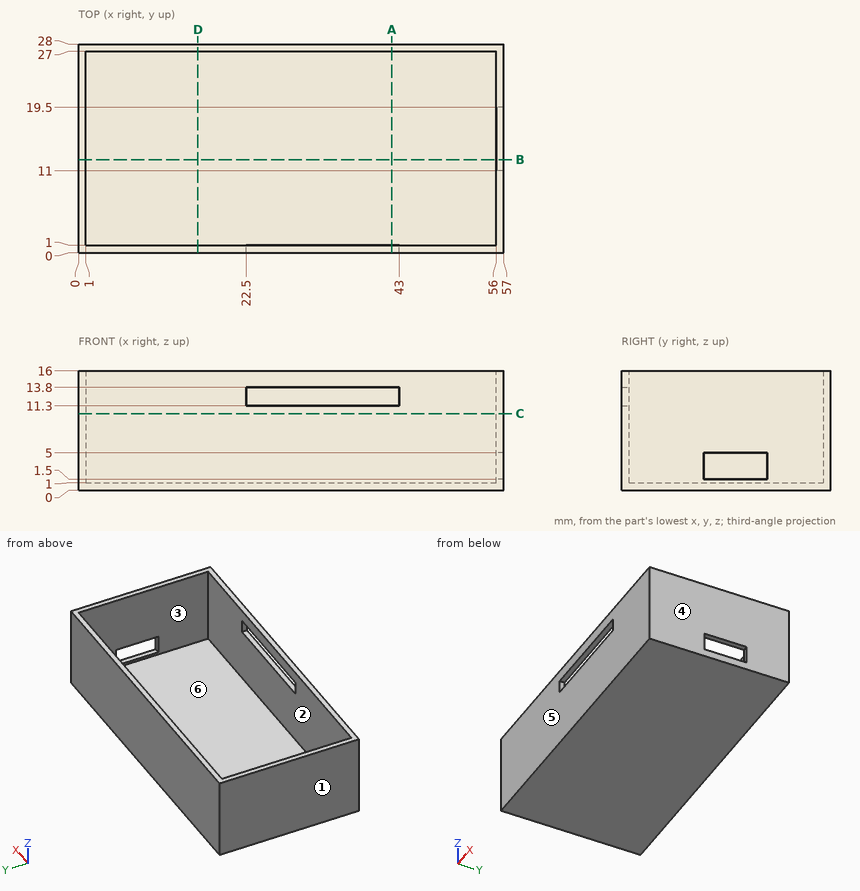
Input: dimensioned drawing with shaded views. Units: mm. Origin: part minimum x, y, z. A direction names the side the tool comes from. Coordinates: 2 decimals unless noted, no trailing zeros. Write each loop counter-clockwise with the first axis right and the second up, starting at its lowest first coordinate (ties: lowest second). Pieces come first, ordered by that corner, then holes. Notation, with made-up numbers: M 47,-6 L 104,-6 A11 cw 104,5 Z; hole C 57,42.25 d4. An arc over 180 degrees is marked long. Use one line per item in the form item = value.
Q1. Section D-D (x = 16). Return loops of the section in (y, z), plus the area to 3 significant figures.
Answer below:
outline = M 0,0 L 28,0 L 28,16 L 27,16 L 27,1 L 1,1 L 1,16 L 0,16 Z
area = 58.0 mm²
Q2. Section C-C (z = 10.25). Return loops of the section in (x, y).
Answer below:
outline = M 0,0 L 57,0 L 57,28 L 0,28 Z; hole M 1,1 L 56,1 L 56,27 L 1,27 Z
Q3. Set-up query: the marked faces 5 and 6. Return all of +Z, -Z, +X, -X, +Y, -Y with unobstructed straight access to the full face (end or side cutting, diameter ignored); none if empty.
Answer below:
face_5 = +Z, -Z, +X, -X, -Y
face_6 = +Z
Q4. Section A-A (x = 42). Return loops of the section in (y, z), plus the area to 3 significant figures.
Answer below:
outline = M 0,0 L 28,0 L 28,16 L 27,16 L 27,1 L 1,1 L 1,11.3 L 0,11.3 Z; M 0,13.8 L 1,13.8 L 1,16 L 0,16 Z
area = 55.5 mm²
Q5. Section B-B (y = 12.5). Return loops of the section in (x, z).
Answer below:
outline = M 0,0 L 57,0 L 57,1.5 L 56,1.5 L 56,1 L 1,1 L 1,16 L 0,16 Z; M 56,5 L 57,5 L 57,16 L 56,16 Z
Q6. Material intervals for probe 1 along X at (y, z) = (17.25, 6.5); probe 2 along Y at (x, z) = (30, 5); probe 3 along Z at (x, y) = (17, 10.25), sorted ascending. Write a range as from..to.
Answer below:
probe_1 = 0..1, 56..57
probe_2 = 0..1, 27..28
probe_3 = 0..1
Q7. Draft query along X for the marked faces 1, 2, 3 and 4. Return one class per face: released by +X, released by -X, zero draft, split by the parting line, or undercut.
Answer below:
face_1 = released by -X
face_2 = undercut
face_3 = undercut
face_4 = released by +X
Q8. First-contact query: pin 1 (3 mm diameter, centred on x = 45.5, y = 21, fed in from +Z). Flat tip, straight axial feed; report the tip coordinate or a pass-through.
Answer below:
pin_1 = 1
